from build123d import *

# Parameters (mm, degrees)
SKETCH1_W           = 30
SKETCH1_H           = 266.8
BOSS_EXTRUDE1_DEPTH = 21
SKETCH2_W           = 19
SKETCH2_H           = 28
CUT_EXTRUDE1_DEPTH  = 270.301392495
CUT_EXTRUDE2_DEPTH  = 270.152819045
CUT_EXTRUDE3_DEPTH  = 270.152819045
CUT_EXTRUDE4_DEPTH  = 270.301392495
CUT_EXTRUDE5_DEPTH  = 270.301392495
CUT_EXTRUDE6_DEPTH  = 270.301392495
CUT_EXTRUDE7_DEPTH  = 270.301392495
SKETCH9_W           = 9.5
SKETCH9_H           = 9.5
CUT_EXTRUDE8_DEPTH  = 270.301392495
SKETCH10_W          = 9.5
SKETCH10_H          = 9.5
CUT_EXTRUDE9_DEPTH  = 270.301392495
SKETCH11_W          = 9.5
SKETCH11_H          = 9.5
CUT_EXTRUDE10_DEPTH = 270.301392495
SKETCH12_W          = 9.5
SKETCH12_H          = 9.5
CUT_EXTRUDE11_DEPTH = 270.301392495
SKETCH13_W          = 9.5
SKETCH13_H          = 9.5
CUT_EXTRUDE12_DEPTH = 270.301392495
SKETCH14_W          = 9.5
SKETCH14_H          = 9.5
CUT_EXTRUDE13_DEPTH = 270.301392495
SKETCH15_W          = 9.5
SKETCH15_H          = 9.5
CUT_EXTRUDE14_DEPTH = 270.301392495
SKETCH16_W          = 9.5
SKETCH16_H          = 9.5
CUT_EXTRUDE15_DEPTH = 270.301392495
SKETCH17_W          = 9.5
SKETCH17_H          = 9.5
CUT_EXTRUDE16_DEPTH = 270.301392495
SKETCH18_W          = 9.5
SKETCH18_H          = 9.5
CUT_EXTRUDE17_DEPTH = 270.301392495
SKETCH19_W          = 9.5
SKETCH19_H          = 9.5
CUT_EXTRUDE18_DEPTH = 270.301392495
SKETCH20_W          = 9.5
SKETCH20_H          = 9.5
CUT_EXTRUDE19_DEPTH = 270.301392495
SKETCH21_W          = 9.5
SKETCH21_H          = 9.5
CUT_EXTRUDE20_DEPTH = 270.301392495
SKETCH22_W          = 9.5
SKETCH22_H          = 9.5
CUT_EXTRUDE21_DEPTH = 270.301392495
SKETCH23_W          = 9.5
SKETCH23_H          = 9.5
CUT_EXTRUDE22_DEPTH = 270.301392495
SKETCH24_W          = 9.5
SKETCH24_H          = 9.5
CUT_EXTRUDE23_DEPTH = 270.301392495
SKETCH25_W          = 9.5
SKETCH25_H          = 9.5
CUT_EXTRUDE24_DEPTH = 270.301392495
SKETCH26_W          = 9.5
SKETCH26_H          = 9.5
CUT_EXTRUDE25_DEPTH = 270.301392495
CUT_EXTRUDE26_DEPTH = 270.152819045
FILLET1_R           = 0.005
FILLET2_R           = 2.005


with BuildPart() as part:
    # Sketch1 → Boss-Extrude1 (new body)
    with BuildSketch(Plane(origin=(0, 0, 0), x_dir=(0, 0, -1), z_dir=(1, 0, 0))):
        with Locations((15, 133.4)):
            Rectangle(SKETCH1_W, SKETCH1_H)
    extrude(amount=-BOSS_EXTRUDE1_DEPTH)

    # Sketch2 → Cut-Extrude1 (cut, through all)
    with BuildSketch(Plane(origin=(0, 266.8, 0), x_dir=(-1, 0, 0), z_dir=(0, 1, 0))):
        with Locations((9.5, -16)):
            Rectangle(SKETCH2_W, SKETCH2_H)
    extrude(amount=-CUT_EXTRUDE1_DEPTH, mode=Mode.SUBTRACT)

    # Sketch3 → Cut-Extrude2 (cut, through all)
    with BuildSketch(Plane(origin=(-19, 0, 0), x_dir=(0, 0, -1), z_dir=(1, 0, 0))):
        with BuildLine():
            Line((12, 266.8), (12, 263.75))
            ThreePointArc((12, 263.75), (15, 260.75), (18, 263.75))
            Line((18, 263.75), (18, 266.8))
            Line((18, 266.8), (12, 266.8))
        make_face()
    extrude(amount=-CUT_EXTRUDE2_DEPTH, mode=Mode.SUBTRACT)

    # Sketch4 → Cut-Extrude3 (cut, through all)
    with BuildSketch(Plane(origin=(-19, 0, 0), x_dir=(0, 0, -1), z_dir=(1, 0, 0))):
        with BuildLine():
            Line((18, 0), (18, 3.05))
            ThreePointArc((18, 3.05), (15, 6.05), (12, 3.05))
            Line((12, 3.05), (12, 0))
            Line((12, 0), (18, 0))
        make_face()
    extrude(amount=-CUT_EXTRUDE3_DEPTH, mode=Mode.SUBTRACT)

    # Sketch5 → Cut-Extrude4 (cut, through all)
    with BuildSketch(Plane.ZY.offset(21)):
        with BuildLine():
            Line((-12, 41.5), (-12, 47.5))
            ThreePointArc((-12, 47.5), (-15, 50.5), (-18, 47.5))
            Line((-18, 47.5), (-18, 41.5))
            ThreePointArc((-18, 41.5), (-15, 38.5), (-12, 41.5))
        make_face()
    extrude(amount=-CUT_EXTRUDE4_DEPTH, mode=Mode.SUBTRACT)

    # Sketch6 → Cut-Extrude5 (cut, through all)
    with BuildSketch(Plane.ZY.offset(21)):
        with BuildLine():
            Line((-12, 85.95), (-12, 91.95))
            ThreePointArc((-12, 91.95), (-15, 94.95), (-18, 91.95))
            Line((-18, 91.95), (-18, 85.95))
            ThreePointArc((-18, 85.95), (-15, 82.95), (-12, 85.95))
        make_face()
    extrude(amount=-CUT_EXTRUDE5_DEPTH, mode=Mode.SUBTRACT)

    # Sketch7 → Cut-Extrude6 (cut, through all)
    with BuildSketch(Plane.ZY.offset(21)):
        with BuildLine():
            Line((-12, 130.4), (-12, 136.4))
            ThreePointArc((-12, 136.4), (-15, 139.4), (-18, 136.4))
            Line((-18, 136.4), (-18, 130.4))
            ThreePointArc((-18, 130.4), (-15, 127.4), (-12, 130.4))
        make_face()
    extrude(amount=-CUT_EXTRUDE6_DEPTH, mode=Mode.SUBTRACT)

    # Sketch8 → Cut-Extrude7 (cut, through all)
    with BuildSketch(Plane.ZY.offset(21)):
        with BuildLine():
            Line((-12, 174.85), (-12, 180.85))
            ThreePointArc((-12, 180.85), (-15, 183.85), (-18, 180.85))
            Line((-18, 180.85), (-18, 174.85))
            ThreePointArc((-18, 174.85), (-15, 171.85), (-12, 174.85))
        make_face()
    extrude(amount=-CUT_EXTRUDE7_DEPTH, mode=Mode.SUBTRACT)

    # Sketch9 → Cut-Extrude8 (cut, through all)
    with BuildSketch(Plane.XY):
        with Locations((-8.5, 244.525)):
            Rectangle(SKETCH9_W, SKETCH9_H)
    extrude(amount=-CUT_EXTRUDE8_DEPTH, mode=Mode.SUBTRACT)

    # Sketch10 → Cut-Extrude9 (cut, through all)
    with BuildSketch(Plane.XY):
        with Locations((-8.5, 228.65)):
            Rectangle(SKETCH10_W, SKETCH10_H)
    extrude(amount=-CUT_EXTRUDE9_DEPTH, mode=Mode.SUBTRACT)

    # Sketch11 → Cut-Extrude10 (cut, through all)
    with BuildSketch(Plane.XY):
        with Locations((-8.5, 215.95)):
            Rectangle(SKETCH11_W, SKETCH11_H)
    extrude(amount=-CUT_EXTRUDE10_DEPTH, mode=Mode.SUBTRACT)

    # Sketch12 → Cut-Extrude11 (cut, through all)
    with BuildSketch(Plane.XY):
        with Locations((-8.5, 200.075)):
            Rectangle(SKETCH12_W, SKETCH12_H)
    extrude(amount=-CUT_EXTRUDE11_DEPTH, mode=Mode.SUBTRACT)

    # Sketch13 → Cut-Extrude12 (cut, through all)
    with BuildSketch(Plane.XY):
        with Locations((-8.5, 184.2)):
            Rectangle(SKETCH13_W, SKETCH13_H)
    extrude(amount=-CUT_EXTRUDE12_DEPTH, mode=Mode.SUBTRACT)

    # Sketch14 → Cut-Extrude13 (cut, through all)
    with BuildSketch(Plane.XY):
        with Locations((-8.5, 171.5)):
            Rectangle(SKETCH14_W, SKETCH14_H)
    extrude(amount=-CUT_EXTRUDE13_DEPTH, mode=Mode.SUBTRACT)

    # Sketch15 → Cut-Extrude14 (cut, through all)
    with BuildSketch(Plane.XY):
        with Locations((-8.5, 155.625)):
            Rectangle(SKETCH15_W, SKETCH15_H)
    extrude(amount=-CUT_EXTRUDE14_DEPTH, mode=Mode.SUBTRACT)

    # Sketch16 → Cut-Extrude15 (cut, through all)
    with BuildSketch(Plane.XY):
        with Locations((-8.5, 139.75)):
            Rectangle(SKETCH16_W, SKETCH16_H)
    extrude(amount=-CUT_EXTRUDE15_DEPTH, mode=Mode.SUBTRACT)

    # Sketch17 → Cut-Extrude16 (cut, through all)
    with BuildSketch(Plane.XY):
        with Locations((-8.5, 127.05)):
            Rectangle(SKETCH17_W, SKETCH17_H)
    extrude(amount=-CUT_EXTRUDE16_DEPTH, mode=Mode.SUBTRACT)

    # Sketch18 → Cut-Extrude17 (cut, through all)
    with BuildSketch(Plane.XY):
        with Locations((-8.5, 111.175)):
            Rectangle(SKETCH18_W, SKETCH18_H)
    extrude(amount=-CUT_EXTRUDE17_DEPTH, mode=Mode.SUBTRACT)

    # Sketch19 → Cut-Extrude18 (cut, through all)
    with BuildSketch(Plane.XY):
        with Locations((-8.5, 95.3)):
            Rectangle(SKETCH19_W, SKETCH19_H)
    extrude(amount=-CUT_EXTRUDE18_DEPTH, mode=Mode.SUBTRACT)

    # Sketch20 → Cut-Extrude19 (cut, through all)
    with BuildSketch(Plane.XY):
        with Locations((-8.5, 82.6)):
            Rectangle(SKETCH20_W, SKETCH20_H)
    extrude(amount=-CUT_EXTRUDE19_DEPTH, mode=Mode.SUBTRACT)

    # Sketch21 → Cut-Extrude20 (cut, through all)
    with BuildSketch(Plane.XY):
        with Locations((-8.5, 66.725)):
            Rectangle(SKETCH21_W, SKETCH21_H)
    extrude(amount=-CUT_EXTRUDE20_DEPTH, mode=Mode.SUBTRACT)

    # Sketch22 → Cut-Extrude21 (cut, through all)
    with BuildSketch(Plane.XY):
        with Locations((-8.5, 50.85)):
            Rectangle(SKETCH22_W, SKETCH22_H)
    extrude(amount=-CUT_EXTRUDE21_DEPTH, mode=Mode.SUBTRACT)

    # Sketch23 → Cut-Extrude22 (cut, through all)
    with BuildSketch(Plane.XY):
        with Locations((-8.5, 38.15)):
            Rectangle(SKETCH23_W, SKETCH23_H)
    extrude(amount=-CUT_EXTRUDE22_DEPTH, mode=Mode.SUBTRACT)

    # Sketch24 → Cut-Extrude23 (cut, through all)
    with BuildSketch(Plane.XY):
        with Locations((-8.5, 22.275)):
            Rectangle(SKETCH24_W, SKETCH24_H)
    extrude(amount=-CUT_EXTRUDE23_DEPTH, mode=Mode.SUBTRACT)

    # Sketch25 → Cut-Extrude24 (cut, through all)
    with BuildSketch(Plane.XY):
        with Locations((-8.5, 6.4)):
            Rectangle(SKETCH25_W, SKETCH25_H)
    extrude(amount=-CUT_EXTRUDE24_DEPTH, mode=Mode.SUBTRACT)

    # Sketch26 → Cut-Extrude25 (cut, through all)
    with BuildSketch(Plane.XY):
        with Locations((-8.5, 260.4)):
            Rectangle(SKETCH26_W, SKETCH26_H)
    extrude(amount=-CUT_EXTRUDE25_DEPTH, mode=Mode.SUBTRACT)

    # Sketch27 → Cut-Extrude26 (cut, through all)
    with BuildSketch(Plane(origin=(-19, 0, 0), x_dir=(0, 0, -1), z_dir=(1, 0, 0))):
        with BuildLine():
            Line((12, 225.3), (12, 219.3))
            ThreePointArc((12, 219.3), (15, 216.3), (18, 219.3))
            Line((18, 219.3), (18, 225.3))
            ThreePointArc((18, 225.3), (15, 228.3), (12, 225.3))
        make_face()
    extrude(amount=-CUT_EXTRUDE26_DEPTH, mode=Mode.SUBTRACT)

    # Fillet1
    fillet1_edges = [part.edges().sort_by_distance(p)[0] for p in [
        (-19, 133.4, -2),
    ]]
    fillet(fillet1_edges, radius=FILLET1_R)

    # Fillet2
    fillet2_edges = [part.edges().sort_by_distance(p)[0] for p in [
        (-21, 133.4, 0),
    ]]
    fillet(fillet2_edges, radius=FILLET2_R)


solid = part.part
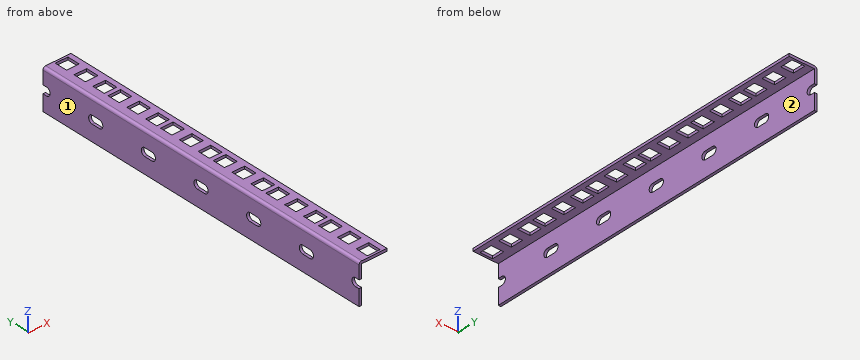
Input: part model. Units: mm. Frame: model coordinates. Face numbers are marked on the shaded views. A direction names the side the tool comes from. Round coordinates to 2 decimals unless told otherwise and drop trailing zeros. Loops run counter-clockwise (first coordinate to the right, second up) from the corner with the lowest first, then second, coordinate; pieces in that order, holes last. Notation, with made-up numbers: (5, 82) -> (25, 82) arc R15 cw to (25, 107) -> close; hole circle Ø5 at (36.5, 57). An arc over 180 degrees is marked (long way). Answer as a JSON object with one key per item and string values. Group by question number.
1) Section query D-D on z = -25.25. Output: boundary loops of the cut face in (x, y).
2) Ray query, L1, parallel to Z at x = -17.25, y = 194; L2, parallel to X at y = 41, z = -20.5; L3, parallel to Z at x = -20, y = 145.5. Return the intervals inside material, ascending.
3) Reachability of the marked faces 1 and 2 from +Z, -Z, +X, -X, +Y, -Y: full face, straight path, thin tool, end or side. Return the list, or none.
4) Pin query (flat end, axial travel): pin 1 (3 mm diameter, centred on x = -12, y = 117.5, fed in from -Z); pin 2 (1.6 mm diameter, centred on x = -20.5, y = 265.5, fed in from +Z); pin 3 (1.6 mm diameter, centred on y = 96, z = -0.5, fed in from -X). Return the tip coordinate at first contact, or that it passes through.
5) Section query A-A on z = -15. Output: boundary loops of the cut face in (x, y).
6) Section query C-C on x = -7.75. State how many separate pieces and enclosed holes the cut face has, plus the area to 3 significant figures.
7) Section query B-B on y = 207.5. Output: boundary loops of the cut face in (x, z) (3 decimals), plus the area to 3 significant figures.
Reply:
{
 "1": {"outline": "(-21, 0) -> (-19, 0) -> (-19, 266.8) -> (-21, 266.8) -> close"},
 "2": {"L1": "z = -2 to 0", "L2": "x = -21 to -19", "L3": "z = -30 to -0.27"},
 "3": {"face 1": "+Z, -Z, -X, +Y, -Y", "face 2": "-Z, +X, +Y, -Y"},
 "4": {"pin 1": "stops at z = -2", "pin 2": "stops at z = -0.13", "pin 3": "stops at x = -20.87"},
 "5": {"outline": "(-21, 6.05) -> (-19, 6.05) -> (-19, 38.5) -> (-21, 38.5) -> close; (-21, 50.5) -> (-19, 50.5) -> (-19, 82.95) -> (-21, 82.95) -> close; (-21, 94.95) -> (-19, 94.95) -> (-19, 127.4) -> (-21, 127.4) -> close; (-21, 139.4) -> (-19, 139.4) -> (-19, 171.85) -> (-21, 171.85) -> close; (-21, 183.85) -> (-19, 183.85) -> (-19, 216.3) -> (-21, 216.3) -> close; (-21, 228.3) -> (-19, 228.3) -> (-19, 260.75) -> (-21, 260.75) -> close"},
 "6": {"separate pieces": "19", "enclosed holes": "0", "area": "192 mm2"},
 "7": {"outline": "(-21, -30) -> (-19, -30) -> (-19, -2.005) arc R0.005 cw to (-18.995, -2) -> (0, -2) -> (0, 0) -> (-18.995, 0) arc R2.005 ccw to (-21, -2.005) -> close", "area": "97.1 mm2"}
}
